Geometry: final body of the model. Coordinates: model frame, mm. Face numbers are marked on the shaded views. A direction names the side the tool comes from. Give positions to 0.01 mm unless a question says otherwise; leave off trailing zeros. Loops run counter-clockwise (first coordinate to the right, second up) from the corner with the lowest first, then second, coordinate; pieces in that order, holes last. Notation, with made-up numbers: (14.25, -28.75) - (44.25, -28.75) arc R28 cw to (44.25, 7.25) - close; hole circle Ø1 at (41, 87). An arc over 180 degrees is marked (long way). Use one line per item in the form item = value.
```python
from build123d import *

# Parameters (mm, degrees)
F0_R     = 9
F1_DEPTH = 10
F4_DEPTH = 200
F6_R     = 9
F7_DEPTH = 10


with BuildPart() as f1:
    # F0 (on Front) → F1 (new body)
    with BuildSketch(Plane.XZ):
        with BuildLine():
            ThreePointArc((-5, 15), (-12.071068, 12.071068), (-15, 5))
            Line((-15, 5), (-15, -64))
            Line((-15, -64), (59, -64))
            Line((59, -64), (59, -20))
            Line((59, -20), (33.445753, -41.98012))
            Line((33.445753, -41.98012), (17, -41.98012))
            ThreePointArc((17, -41.98012), (15.585786, -41.394334), (15, -39.98012))
            Line((15, -39.98012), (15, 5))
            ThreePointArc((15, 5), (12.071068, 12.071068), (5, 15))
            Line((5, 15), (-5, 15))
        make_face()
        Circle(F0_R, mode=Mode.SUBTRACT)
    extrude(amount=-F1_DEPTH)

    # F3 (on offset) → F4 (join)
    with BuildSketch(Plane.XZ.offset(-10)):
        with BuildLine():
            Line((6, -60.5), (6, -61))
            Line((6, -61), (56, -61))
            Line((56, -61), (56, -41))
            Line((56, -41), (55.5, -41))
            ThreePointArc((55.5, -41), (53.732233, -41.732233), (53, -43.5))
            Line((53, -43.5), (53, -53))
            ThreePointArc((53, -53), (51.535534, -56.535534), (48, -58))
            Line((48, -58), (8.5, -58))
            ThreePointArc((8.5, -58), (6.732233, -58.732233), (6, -60.5))
        make_face()
    extrude(amount=-F4_DEPTH)

    # F6 (on offset) → F7 (join)
    with BuildSketch(Plane.XZ.offset(-210)):
        with BuildLine():
            ThreePointArc((-5, 15), (-12.071068, 12.071068), (-15, 5))
            Line((-15, 5), (-15, -64))
            Line((-15, -64), (59, -64))
            Line((59, -64), (59, -20))
            Line((59, -20), (33.445753, -41.98012))
            Line((33.445753, -41.98012), (17, -41.98012))
            ThreePointArc((17, -41.98012), (15.585786, -41.394334), (15, -39.98012))
            Line((15, -39.98012), (15, 5))
            ThreePointArc((15, 5), (12.071068, 12.071068), (5, 15))
            Line((5, 15), (-5, 15))
        make_face()
        Circle(F6_R, mode=Mode.SUBTRACT)
    extrude(amount=-F7_DEPTH)


solid = f1.part
```
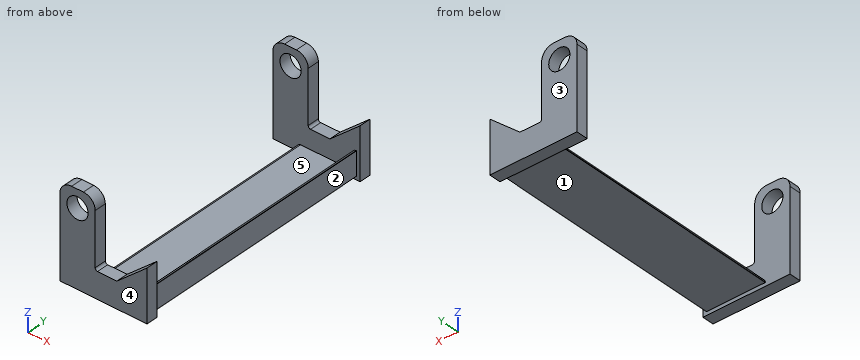
(1) Cut plane B-B (x = 0). Return the cut outline in (y, z), plus the area to 3 significant figures.
Solution:
outline = (0, -64) - (10, -64) - (10, -9) - (0, -9) - close; (0, 9) - (10, 9) - (10, 15) - (0, 15) - close; (210, -64) - (220, -64) - (220, -9) - (210, -9) - close; (210, 9) - (220, 9) - (220, 15) - (210, 15) - close
area = 1,220 mm2
(2) Pull-direction query (Y, two-part tool) for the marked faces 3, 4 and 5; classes: released by +Y, released by -Y, zero draft, split by the parting line, or undercut.
Solution:
face_3 = released by +Y
face_4 = released by -Y
face_5 = undercut
(3) Access query for the marked faces 1 and 2. Directions: +Z, -Z, +X, -X, +Y, -Y. A direction counts if a zero-diameter tool reaches every point of the face in a straight line with its end or side. Return the directions, or none.
Solution:
face_1 = -Z, +X, -X
face_2 = +Z, -Z, +X
(4) Material intervals for L1, parallel to Y at x = 1, z = -38.5; L2, parallel to Z at x = 0, y = 213.5; L3, parallel to Z at x = 47, y = 97, sorted ascending. Write a range as from..to.
Solution:
L1 = 0..10, 210..220
L2 = -64..-9, 9..15
L3 = -61..-58
(5) Cut plane C-C (y = 70.5). Return the cut outline in (x, z), plus the area to 3 significant figures.
Solution:
outline = (6, -61) - (56, -61) - (56, -41) - (55.5, -41) arc R2.5 ccw to (53, -43.5) - (53, -53) arc R5 cw to (48, -58) - (8.5, -58) arc R2.5 ccw to (6, -60.5) - close
area = 204 mm2
(6) Cut plane A-A (z = 0). Return the cut outline in (x, y), plus the area to 3 significant figures.
Solution:
outline = (-15, 0) - (-9, 0) - (-9, 10) - (-15, 10) - close; (-15, 210) - (-9, 210) - (-9, 220) - (-15, 220) - close; (9, 0) - (15, 0) - (15, 10) - (9, 10) - close; (9, 210) - (15, 210) - (15, 220) - (9, 220) - close
area = 240 mm2
(7) Pin query (flat end, axial travel): P1, Ø16, axis at y = 97, z = -52, coming from the +X side; P2, Ø4, axis at x = 41, z = -37, coming from the -Y side; P3, Ø0.6, axis at y = 96.5, z = -60.5, coming from the -X side; P4, Ø15, axis at x = 30, y = 107.5, coming from the -Z side. Return the tip coordinate at first contact, or that it passes through.
Solution:
P1 = 56
P2 = 0
P3 = 6
P4 = -61
(8) Cut plane D-D (z = -12.5). Return the cut outline in (x, y).
Solution:
outline = (-15, 0) - (15, 0) - (15, 10) - (-15, 10) - close; (-15, 210) - (15, 210) - (15, 220) - (-15, 220) - close
